Build history of the part. All positions in model axes, mm. A direction names the side the tool comes from. Round coordinates to 2 decimals unless told otherwise and drop trailing zeros. Loops run counter-clockwise (first coordinate to the right, second up) from the corner with the lowest first, then second, coordinate; pieces in that order, holes last.
from build123d import *

# Parameters (mm, degrees)
ESBO_O1_R                                    = 10.5
RESSALTO_EXTRUS_O1_DEPTH                     = 124
FILETE1_R                                    = 1
BROCA_DE_ROSQUEAR_PARA_TARRAXA_DE_M101_D     = 8.5
BROCA_DE_ROSQUEAR_PARA_TARRAXA_DE_M101_DEPTH = 25
BROCA_DE_ROSQUEAR_PARA_TARRAXA_DE_M101_TIP   = 2.553657631
BROCA_DE_ROSQUEAR_PARA_TARRAXA_DE_M102_D     = 8.5
BROCA_DE_ROSQUEAR_PARA_TARRAXA_DE_M102_DEPTH = 25
BROCA_DE_ROSQUEAR_PARA_TARRAXA_DE_M102_TIP   = 2.553657631


with BuildPart() as part:
    # Esboço1 → Ressalto-extrusão1 (new body)
    with BuildSketch(Plane.XY):
        with Locations((-70, 54)):
            Circle(ESBO_O1_R)
    extrude(amount=-RESSALTO_EXTRUS_O1_DEPTH)

    # Filete1
    filete1_edges = [part.edges().sort_by_distance(p)[0] for p in [
        (-80.5, 54, 0),
        (-80.5, 54, -124),
    ]]
    fillet(filete1_edges, radius=FILETE1_R)

    # Broca de rosquear para tarraxa de M101
    with Locations(Plane.XY):
        with Locations((-70, 54)):
            Hole(BROCA_DE_ROSQUEAR_PARA_TARRAXA_DE_M101_D / 2, depth=BROCA_DE_ROSQUEAR_PARA_TARRAXA_DE_M101_DEPTH)
            with Locations((0, 0, -(BROCA_DE_ROSQUEAR_PARA_TARRAXA_DE_M101_DEPTH + BROCA_DE_ROSQUEAR_PARA_TARRAXA_DE_M101_TIP / 2))):  # 118° drill point
                Cone(0, BROCA_DE_ROSQUEAR_PARA_TARRAXA_DE_M101_D / 2, BROCA_DE_ROSQUEAR_PARA_TARRAXA_DE_M101_TIP, mode=Mode.SUBTRACT)

    # Broca de rosquear para tarraxa de M102
    with Locations(Plane(origin=(0, 0, -124), x_dir=(-1, 0, 0), z_dir=(0, 0, -1))):
        with Locations((70, 54)):
            Hole(BROCA_DE_ROSQUEAR_PARA_TARRAXA_DE_M102_D / 2, depth=BROCA_DE_ROSQUEAR_PARA_TARRAXA_DE_M102_DEPTH)
            with Locations((0, 0, -(BROCA_DE_ROSQUEAR_PARA_TARRAXA_DE_M102_DEPTH + BROCA_DE_ROSQUEAR_PARA_TARRAXA_DE_M102_TIP / 2))):  # 118° drill point
                Cone(0, BROCA_DE_ROSQUEAR_PARA_TARRAXA_DE_M102_D / 2, BROCA_DE_ROSQUEAR_PARA_TARRAXA_DE_M102_TIP, mode=Mode.SUBTRACT)


solid = part.part
(1) Pin check, flat tips, straight feed: P1, Ø5, axis at x = -70, y = 54, coming from the -Z side; P2, Ø1.5, axis at x = -65.5, z = -97.5, coming from the -Y side; P3, Ø3, axis at y = 60.5, z = -19.5, coming from the -X side. Stop position of each tip, or through.
Responses:
P1: stops at z = -97.95
P2: stops at y = 44.19
P3: stops at x = -79.23
(2) Slice it at A-A on z = -113.5. List the corners of the cut face in (x, y), plus the area to 3 significant figures.
Responses:
outline: circle Ø21 at (-70, 54); hole circle Ø8.5 at (-70, 54)
area: 290 mm2
(3) Probe line 1 (Y direction, x = -70, z = -110.75); line 2 (Y direction, x = -72.25, z = -6); line 3 (Z direction, x = -63.25, y = 47.25). List the from-to ranges inside material, lowest first.
Responses:
line 1: y = 43.5 to 49.75, 58.25 to 64.5
line 2: y = 43.74 to 50.39, 57.61 to 64.26
line 3: z = -124 to 0
(4) Slice it at B-B on z = -75.5. List the corners of the cut face in (x, y).
Responses:
outline: circle Ø21 at (-70, 54)
(5) Pull direction Y, two halves, no side cores. Call faces 1 (the face through (-66, 52, -124)), 2 (the face through (-69.46, 54.5, -96.89)), 3 (the face through (-78.33, 47.61, -61.15)): +Y half, -Y half, draft (parallel to the pull), parting line (faces both ways), or undercut.
Responses:
face 1: draft
face 2: undercut
face 3: parting line
(6) Which spindle directions (+Z, -Z, +X, -X, +Y, -Y) get a long thin tool onto all of the face, cutting with end or side? Do faces 4 (the face through (-68.04, 50.23, -111.32)), 5 (the face through (-71.96, 50.23, -12.67)), 6 (the face through (-66, 52, 0)). Say none if no direction does.
Responses:
face 4: -Z
face 5: +Z
face 6: +Z, +X, -X, +Y, -Y
